Part model, mm, in its own coordinate system. Round coordinates to 2 decimals unless told otherwise and drop trailing zeros. Write each loop counter-clockwise with the first axis right and the second up, starting at its lowest first coordinate (ties: lowest second). Pieces come first, ordered by that corner, then holes. Notation, with made-up numbers: M 82.5,-17.5 L 137.5,-17.5 A10 cw 137.5,-4.5 Z; hole C -2.75,-36 d1. An arc over 180 degrees is marked long. Answer as a JSON object with one key per item and string values. Group by question number.
1. Drop flat-ended pins along their axis: pin 1 (2 mm diameter, centred on y = -13.5, z = 85, fed in from +X); pin 2 (5 mm diameter, centred on x = -10.5, z = 142, fed in from -Y); pin 3 (5 mm diameter, centred on x = -8, z = 83.5, fed in from -Y); pin 4 (10 mm diameter, centred on x = 1, y = -15.5, fed in from -Z). Give the stop position or say it passes through.
2. Band-saw the part on A-A, the plane z = 157. Write the cut outline in (x, y), plus the area to 3 significant figures.
3. Drill centre lines: line 1 (X direction, y = 4, z = 95.5); line 2 (Y direction, x = -13.5, z = 10.5); line 3 (X direction, y = -11, z = 169.5). Where is each one in solid material? Low to high. Write a range as from..to.
4. Band-saw the part on B-B, the plane x = 13. Write the cut outline in (y, z).
5. Band-saw the part on C-C, the plane y = 6. Write the cut outline in (x, z), plus the area to 3 significant figures.
from build123d import *

# Parameters (mm, degrees)
F0_R      = 25
F0_R_2    = 24.25
F1_DEPTH  = 180
F2_W      = 6.5743785797
F2_H      = 144
F2_W_2    = 7.4769609538
F3_DEPTH  = 1.5
F4_DEPTH  = 4
F5_DEPTH  = 4
F6_W      = 7.290615557
F6_H      = 144
F6_W_2    = 7.1577106116
F7_DEPTH  = 1.5
F8_DEPTH  = 4
F9_DEPTH  = 25
F10_DEPTH = 10


# Not quite as in the source:
# - a feature names something its author has since deleted; it is built from what else it names


with BuildPart() as f1:
    # F0 (on Top) → F1 (new body)
    with BuildSketch(Plane.XY):
        Circle(F0_R)
        Circle(F0_R_2, mode=Mode.SUBTRACT)
    extrude(amount=F1_DEPTH)

    # F2 (on Right) → F3 (cut, symmetric)
    with BuildSketch(Plane.YZ):
        with Locations((-28.224690467, 88)):
            Rectangle(F2_W, F2_H)
        with Locations((28.6692082882, 88)):
            Rectangle(F2_W_2, F2_H)
    extrude(amount=F3_DEPTH, both=True, mode=Mode.SUBTRACT)

    # F4 (cut): faces of the model
    f4_faces = [f1.faces().sort_by_distance(p)[0] for p in [
        (0, -24.9375011772, 88),
        (0, 24.9307278113, 88),
    ]]
    extrude(f4_faces, amount=-F4_DEPTH, dir=(0, -1, 0), mode=Mode.SUBTRACT)

    # F5 (cut): a face of the model
    f5_faces = [f1.faces().sort_by_distance(p)[0] for p in [
        (0, 24.9307278113, 88),
    ]]
    extrude(f5_faces, amount=-F5_DEPTH, mode=Mode.SUBTRACT)

    # F6 (on Front) → F7 (join, symmetric)
    with BuildSketch(Plane.XZ):
        with Locations((28.4072192601, 88)):
            Rectangle(F6_W, F6_H)
        with Locations((-28.2881861775, 88)):
            Rectangle(F6_W_2, F6_H)
    extrude(amount=F7_DEPTH, both=True)

    # F8 (cut): faces of the model
    f8_faces = [f1.faces().sort_by_distance(p)[0] for p in [
        (32.0525270386, 0, 88),
        (-31.8670414833, 0, 88),
    ]]
    extrude(f8_faces, amount=-F8_DEPTH, dir=(1, 0, 0), mode=Mode.SUBTRACT)

    # F9 (cut): a face of the model
    f9_faces = [f1.faces().sort_by_distance(p)[0] for p in [
        (28.0525270386, 0, 88),
    ]]
    extrude(f9_faces, amount=-F9_DEPTH, mode=Mode.SUBTRACT)

    # F10 (cut): a face of the model
    f10_faces = [f1.faces().sort_by_distance(p)[0] for p in [
        (-31.8670414833, 0, 88),
    ]]
    extrude(f10_faces, amount=-F10_DEPTH, mode=Mode.SUBTRACT)


solid = f1.part
Worked answers:
{
 "1": {"pin 1": "stops at x = 21.65", "pin 2": "stops at y = -23.69", "pin 3": "stops at y = -24.39", "pin 4": "passes through"},
 "2": {"outline": "M -24.95,-1.5 A25 ccw -1.5,-24.95 L -1.5,-24.2 A24.25 cw -24.2,-1.5 Z; M -24.95,1.5 L -24.2,1.5 A24.25 cw -1.5,24.2 L -1.5,24.95 A25 ccw Z; M 1.5,-24.95 A25 ccw 24.95,-1.5 L 24.2,-1.5 A24.25 cw 1.5,-24.2 Z; M 1.5,24.2 A24.25 cw 24.2,1.5 L 24.95,1.5 A25 ccw 1.5,24.95 Z", "area": "107 mm^2"},
 "3": {"line 1": "x = -24.68..-23.92, 23.92..24.68", "line 2": "y = -21.04..-20.14, 20.14..21.04", "line 3": "x = -22.45..-21.61, 21.61..22.45"},
 "4": {"outline": "M -21.35,0 L -20.47,0 L -20.47,180 L -21.35,180 Z; M 20.47,0 L 21.35,0 L 21.35,180 L 20.47,180 Z"},
 "5": {"outline": "M -24.27,0 L -23.5,0 L -23.5,180 L -24.27,180 Z; M 23.5,0 L 24.27,0 L 24.27,180 L 23.5,180 Z", "area": "278 mm^2"}
}
